CAD build for the part. Positions are in the model's coordinates, mm. A direction names the side the tool comes from. Round coordinates to 2 decimals unless told otherwise and drop trailing zeros. Write each loop counter-clockwise with the first axis right and the second up, starting at its lowest first coordinate (ties: lowest second). Pieces come first, ordered by that corner, then holes. Notation, with made-up numbers: (-4.75, 19.5) - (10.25, 19.5) arc R18 ccw to (10.25, 34.5) - close; hole circle Ø7 at (54.5, 71). An arc over 180 degrees is marked (long way). Use one line per item in the form item = value. Start each with the question number.
Item 1: Drill centre lines: L1, parallel to X at y = -1.05, z = 108; L2, parallel to Z at x = 0.5, y = -1.7; L3, parallel to X at y = -1.1, z = 56.5. Where is each one in solid material? Low to high.
Item 2: Tool access for faces 1 (the flat face through (32, -2, 49)), 2 (the flat face through (-29.767, -0.986, 34.434)): list every direction of +Z, -Z, +X, -X, +Y, -Y with a clear straight run to the whole face (end or side of a thin tool).
Item 3: Band-saw the part on C-C, the plane z = 36. List the corners of the cut face in (x, y).
Item 4: Pull direction X, two halves, no side cores. Call faces 3 (the flat face through (32, 0, 49)), 4 (the flat face through (29.767, -0.986, 34.434)), 5 (the flat face through (-32.465, -0.986, 30.566)): +X half, -X half, draft (parallel to the pull), parting line (faces both ways), or undercut.
Item 5: Band-saw the part on B-B, the plane y = -1. List the corners of the cut face in (x, z).
Item 6: Band-saw the part on A-A, the plane z = 76. List the corners of the cut face in (x, y).
Item 7: Pin check, flat tips, straight feed: pin 1 (1 mm diameter, centred on x = -37.5, y = -1, fed in from +Z); pin 2 (1 mm diameter, centred on x = 40, y = -0.5, fed in from -Z). Stop position of each tip, or through.
Item 8: Band-saw the part on D-D, the plane x = 2.5. List the corners of the cut face in (y, z), and give its area (3 significant figures).
from build123d import *

# Parameters (mm, degrees)
F1_DEPTH = 2


with BuildPart() as f1:
    # F0 (on Front) → F1 (new body)
    with BuildSketch(Plane.XZ):
        Polygon((0, 3), (0, 0), (30, 0), (35, 62), (43, 62), (43, 125), (40, 125), (40, 65), (32.232196, 65), (27.232196, 3), align=None)
    extrude(amount=F1_DEPTH)

    # F2: F1 across plane


with BuildPart() as f1_1:
    add(f1.part)
    add(f1.part.mirror(Plane.YZ))


solid = f1_1.part
Determined:
q1.L1 = -43 to -40, 40 to 43
q1.L2 = 0 to 3
q1.L3 = -34.56 to -31.55, 31.55 to 34.56
q2.face_1 = +Z, -Z, +X, -X, -Y
q2.face_2 = +Z, +Y, -Y
q3.outline = (-32.9, -2) - (-29.89, -2) - (-29.89, 0) - (-32.9, 0) - close; (29.89, -2) - (32.9, -2) - (32.9, 0) - (29.89, 0) - close
q4.face_3 = draft
q4.face_4 = undercut
q4.face_5 = -X half
q5.outline = (-43, 62) - (-35, 62) - (-30, 0) - (30, 0) - (35, 62) - (43, 62) - (43, 125) - (40, 125) - (40, 65) - (32.23, 65) - (27.23, 3) - (-27.23, 3) - (-32.23, 65) - (-40, 65) - (-40, 125) - (-43, 125) - close
q6.outline = (-43, -2) - (-40, -2) - (-40, 0) - (-43, 0) - close; (40, -2) - (43, -2) - (43, 0) - (40, 0) - close
q7.pin_1 = 65
q7.pin_2 = 62
q8.outline = (-2, 0) - (0, 0) - (0, 3) - (-2, 3) - close
q8.area = 6.00 mm²
